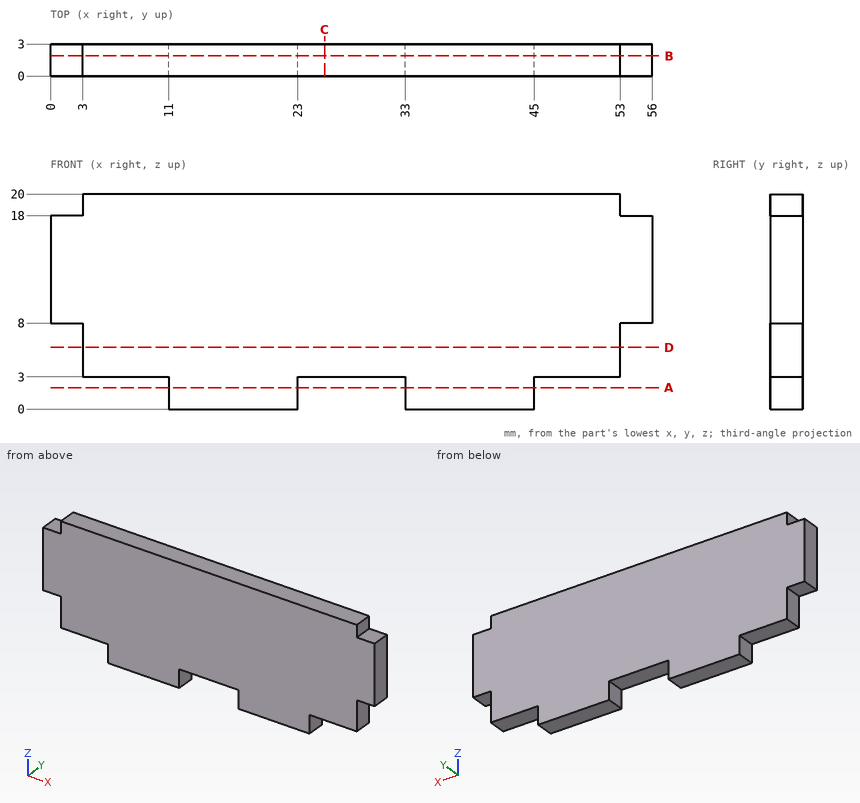
For this review, use the dimensioned drawing (mm, ordinates from the lowest corner) and the shaded views. Coordinates: 2 decimals unless noted, no trailing zeros. Write each loop counter-clockwise with the first axis right and the second up, starting at its lowest first coordinate (ties: lowest second). Pieces come first, ordered by that corner, then holes. Notation, with made-up numbers: (-17, 25.5) - (6, 25.5) arc R30 cw to (6, 58.5) - close; hole circle Ø2 at (30, 52.5). An arc over 180 degrees is marked (long way). Answer as a JSON object with one key per item and string values. Group by question number.
1. Add section A-A (z = 2). Give the boundary of the cut face in (x, y), plus the area to 3 significant figures.
2. Clearance check with flat-ended pins moving along their axes: pin 1 Ø0.9 at (y, z) = (2, 6.5) entering from -X; pin 2 Ø1.5 at (y, z) = (1, 1.5) entering from +X; pin 3 Ø0.9 at (x, y) = (29, 1.5) entering from -Z. State where each tip first meets the part, or that it passes through.
3. Add section C-C (x = 25.5). Give the boundary of the cut face in (y, z), plus the area to 3 significant figures.
4. Add section D-D (z = 5.75). Give the boundary of the cut face in (x, y), plus the area to 3 significant figures.
5. To check wall thickness, follow probe 1 along X at (y, z) = (1.3, 1.25); probe 2 along Z at (x, y) = (49, 2.7); probe 3 along X at (y, z) = (0.4, 19). State the ranges of each line that lie inside material, in increasing order.
6. Add section B-B (y = 1.9). Give the boundary of the cut face in (x, z), plus the area to 3 significant figures.
Findings:
{
 "1": {"outline": "(11, 0) - (23, 0) - (23, 3) - (11, 3) - close; (33, 0) - (45, 0) - (45, 3) - (33, 3) - close", "area": "72.0 mm²"},
 "2": {"pin 1": "x = 3", "pin 2": "x = 45", "pin 3": "z = 3"},
 "3": {"outline": "(0, 3) - (3, 3) - (3, 20) - (0, 20) - close", "area": "51.0 mm²"},
 "4": {"outline": "(3, 0) - (53, 0) - (53, 3) - (3, 3) - close", "area": "150 mm²"},
 "5": {"probe 1": "11 to 23, 33 to 45", "probe 2": "3 to 20", "probe 3": "3 to 53"},
 "6": {"outline": "(0, 8) - (3, 8) - (3, 3) - (11, 3) - (11, 0) - (23, 0) - (23, 3) - (33, 3) - (33, 0) - (45, 0) - (45, 3) - (53, 3) - (53, 8) - (56, 8) - (56, 18) - (53, 18) - (53, 20) - (3, 20) - (3, 18) - (0, 18) - close", "area": "982 mm²"}
}
